Input: dimensioned drawing with shaded views. Units: mm. Origin: part minimum x, y, z. Give positions to 0.01 mm unless a question says otherwise; leave off trailing zeros. Write each loop counter-clockwise with the first axis right and the second up, starting at its lowest first coordinate (ties: lowest second). Pieces come first, ordered by that corner, then holes.
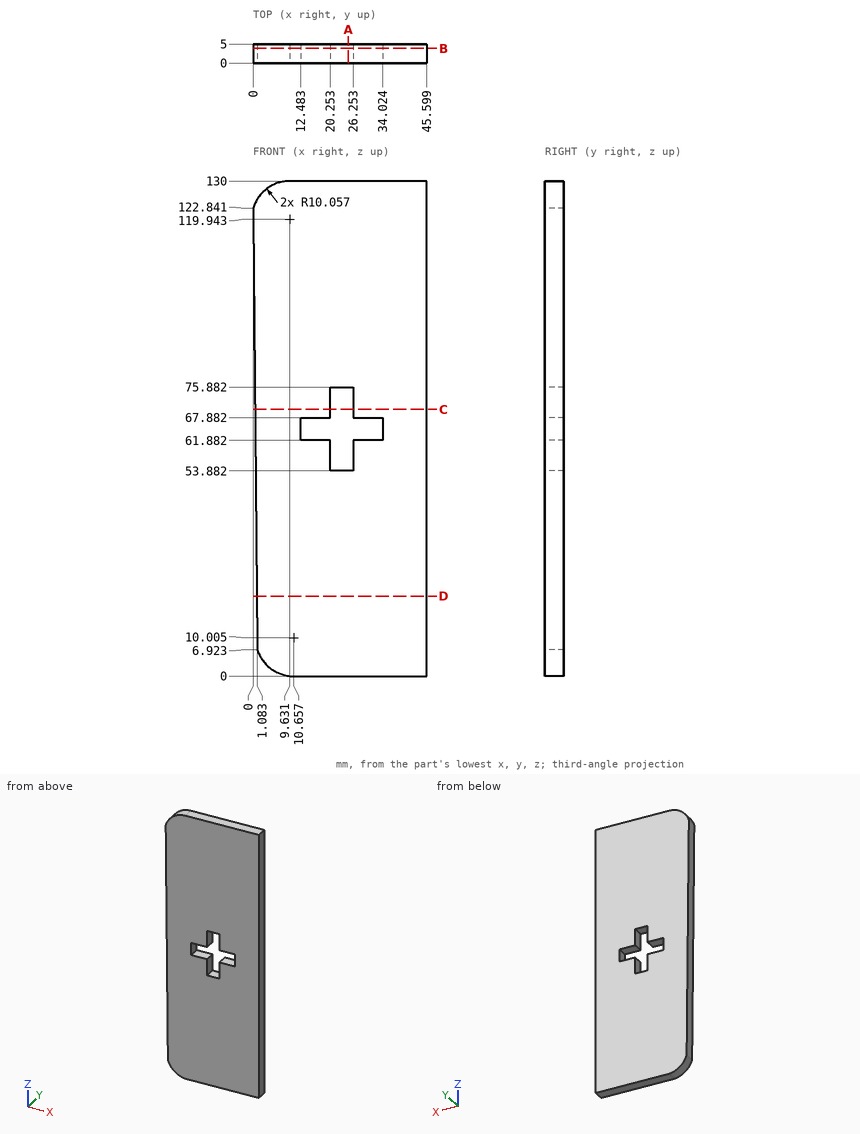
Item 1: Line query: L1, parallel to Z at x = 26.5, y = 3.5; L2, parallel to Z at x = 9.5, y = 1.75 (1 decimal); L3, parallel to X at y = 4.4, z = 57.5. Output: solid intervals per line, ascending.
Found:
L1: z = 0 to 61.88, 67.88 to 130
L2: z = 0 to 130
L3: x = 0.61 to 20.25, 26.25 to 45.6
Item 2: Pin query (flat end, axial travel): pin 1 Ø2.5 at (y, z) = (3.5, 60) entering from -X (1 decimal); pin 2 Ø1.5 at (x, y) = (15.5, 2) entering from -Z; pin 3 Ø2.5 at (y, z) = (3, 64.5) entering from -X; pin 4 Ø2 at (y, z) = (2, 16.5) entering from -X. Return the tip coordinate at first contact, or that it passes through.
Found:
pin 1: stops at x = 0.6
pin 2: stops at z = 0
pin 3: stops at x = 0.53
pin 4: stops at x = 0.98
Item 3: Section A-A, the plane x = 25. Return the cut outline in (y, z).
Found:
outline: (0, 0) - (5, 0) - (5, 53.88) - (0, 53.88) - close; (0, 75.88) - (5, 75.88) - (5, 130) - (0, 130) - close
Item 4: Section C-C, the plane z = 70. Return the cut outline in (x, y).
Found:
outline: (0.49, 0) - (20.25, 0) - (20.25, 5) - (0.49, 5) - close; (26.25, 0) - (45.6, 0) - (45.6, 5) - (26.25, 5) - close
Item 5: Section D-D, the plane z = 21. Return the cut outline in (x, y), plus the area to 3 significant figures.
Found:
outline: (0.95, 0) - (45.6, 0) - (45.6, 5) - (0.95, 5) - close
area: 223 mm2
Item 6: Section B-B, the plane y = 3.85. Return the cut outline in (x, z) (1 decimal), plus the area to 3 significant figures.
Found:
outline: (0, 122.8) - (1.1, 6.9) arc R10.1 ccw to (9.6, 0) - (45.6, 0) - (45.6, 130) - (9.6, 130) arc R10.1 ccw to start; hole (12.5, 61.9) - (20.3, 61.9) - (20.3, 53.9) - (26.3, 53.9) - (26.3, 61.9) - (34, 61.9) - (34, 67.9) - (26.3, 67.9) - (26.3, 75.9) - (20.3, 75.9) - (20.3, 67.9) - (12.5, 67.9) - close
area: 5,600 mm2
